The listing builds one solid part. Answer for the finished solid, in the listing's coordinates (mm). A direction names the side the tool comes from. Give positions to 0.01 mm unless a question says otherwise; leave off trailing zeros. Write each loop counter-clockwise with the first axis right and the second up, starting at its lowest first coordinate (ties: lowest second). Pieces come first, ordered by that corner, then holes. Notation, with made-up numbers: (44.25, 44) -> (92.25, 44) arc R18 cw to (92.25, 72) -> close; hole circle Ø3 at (69.5, 74). An arc over 180 degrees is marked (long way). Write each question's results on one line, items separated by ' | '. Start each with the question number.
from build123d import *

# Parameters (mm, degrees)
CUT_EXTRUDE2_DEPTH      = 20
CUT_EXTRUDE3_START      = -20
SKETCH8_R               = 5
CUT_EXTRUDE3_DEPTH      = 20
CUT_EXTRUDE4_DEPTH      = 43.426406871
CUT_EXTRUDE4_DEPTH_BACK = 43.426406871
SKETCH11_R              = 0.7
CUT_EXTRUDE5_DEPTH      = 30.669007398
SKETCH13_R              = 1.3
CUT_EXTRUDE6_DEPTH      = 4


with BuildPart() as part:
    # Sketch5 → Revolve2 (revolve)
    with BuildSketch(Plane.XY, mode=Mode.PRIVATE) as revolve2_sk:
        Polygon((-9.041219405, 20), (0, 20), (0, -20), (-9.041219405, -20), (-10, -19), (-10, -1), (-9.041219405, 0), (-10, 1), (-10, 19), align=None)
    revolve(revolve2_sk.sketch.rotate(Axis((0, -53.191489362, 0), (0, 1, 0)), 180), axis=Axis((0, -53.191489362, 0), (0, 1, 0)))

    # Sketch6 → Cut-Extrude2 (cut)
    with BuildSketch(Plane(origin=(0, -20, 0), x_dir=(-1, 0, 0), z_dir=(0, -1, 0))):
        with BuildLine():
            Line((-3, 4), (-3, -4))
            ThreePointArc((-3, -4), (0, -5), (3, -4))
            Line((3, -4), (3, 4))
            ThreePointArc((3, 4), (0, 5), (-3, 4))
        make_face()
    extrude(amount=-CUT_EXTRUDE2_DEPTH, mode=Mode.SUBTRACT)

    # Sketch8 → Cut-Extrude3 (cut)
    with BuildSketch(Plane(origin=(0, 20, 0), x_dir=(1, 0, 0), z_dir=(0, 1, 0)).offset(CUT_EXTRUDE3_START)):
        with Locations(Location((0, 0, 0), (0, 0, 306.869897646))):
            Circle(SKETCH8_R)
    extrude(amount=CUT_EXTRUDE3_DEPTH, mode=Mode.SUBTRACT)

    # Sketch9 → Cut-Extrude4 (cut, two sides: drawn at the far end of the back side and taken through both)
    with BuildSketch(Plane(origin=(0, 20, 0), x_dir=(1, 0, 0), z_dir=(0, 1, 0)).offset(-CUT_EXTRUDE4_DEPTH_BACK)):
        with BuildLine():
            Line((-0.5, -4.974937186), (-0.5, -10.403800493))
            ThreePointArc((-0.5, -10.403800493), (0, -10.415808404), (0.5, -10.403800493))
            Line((0.5, -10.403800493), (0.5, -4.974937186))
            ThreePointArc((0.5, -4.974937186), (0, -5), (-0.5, -4.974937186))
        make_face()
    extrude(amount=CUT_EXTRUDE4_DEPTH + CUT_EXTRUDE4_DEPTH_BACK, mode=Mode.SUBTRACT)

    # Sketch11 → Cut-Extrude5 (cut, through all)
    with BuildSketch(Plane(origin=(9.5, 0, 0), x_dir=(0, 0, -1), z_dir=(1, 0, 0))):
        with Locations(Location((-7.5, 15, 0), (0, 0, 90))):
            Circle(SKETCH11_R)
        with Locations(Location((-7.5, 5, 0), (0, 0, 90))):
            Circle(SKETCH11_R)
        with Locations(Location((-7.5, -5, 0), (0, 0, 90))):
            Circle(SKETCH11_R)
        with Locations(Location((-7.5, -15, 0), (0, 0, 90))):
            Circle(SKETCH11_R)
    extrude(amount=-CUT_EXTRUDE5_DEPTH, mode=Mode.SUBTRACT)

    # Sketch13 → Cut-Extrude6 (cut)
    with BuildSketch(Plane(origin=(9.5, 0, 0), x_dir=(0, 0, -1), z_dir=(1, 0, 0))):
        with Locations((-7.5, 15)):
            Circle(SKETCH13_R)
        with Locations((-7.5, 5)):
            Circle(SKETCH13_R)
        with Locations((-7.5, -5)):
            Circle(SKETCH13_R)
        with Locations((-7.5, -15)):
            Circle(SKETCH13_R)
    extrude(amount=-CUT_EXTRUDE6_DEPTH, mode=Mode.SUBTRACT)


solid = part.part
1. The mould has two halves that part along Z. Classify faces 5 (the flat face through (-0.5, 0, 7)), 6 (the cylindrical face through (3.04, 4.48, 7.97)): pulls with the +Z half, pulls with the -Z half, needs draft (parallel to the pull), parting line crosses it, or undercut.
2. Section C-C (y = -9) is taken. Write down the section's boundary in (x, z).
3. Consider probe 1 along Y at (x, z) = (-3.75, 7.5); probe 2 along Y at (x, z) = (6.55, 7.5); probe 3 along Z at (x, y) = (1.5, -15). Determine where each line is inside the solid, lowest interval first. Write a range as [from, to].
4. Section D-D (x = -4) is taken. Give the number of separate pieces and of enclosed holes in the cut face, then the cut area to 3 significant figures.
5. Each of these flat-tipped pins is pushed along its axis until it touches: pin 1 Ø0.8 at (y, z) = (-15, 7.5) entering from -X; pin 2 Ø2 at (y, z) = (-5, 7.5) entering from +X; pin 3 Ø1 at (x, y) = (7, -10) entering from +Z; pin 4 Ø4 at (y, z) = (-15, 7.5) entering from -X. Where does it stop, or does it pass through?
6. Section A-A (y = -15) is taken. Write down the section's boundary in (x, z).
7. A tool of negligible diameter and unlimited length cuts with its end or side. For faces 1 (the flat face through (0.5, 0, 8)), 2 (the flat face through (4, 0, 0)), 3 (the cylindrical face through (6.4, 15, 6.2)), 4 (the flat face through (3, -10, 0)), from which of +Z, -Z, +X, -X, +Y, -Y can it reach the whole face along a straight path? Write none if from no direction.
8. Section B-B (x = 0) is taken. Write down the section's boundary in (y, z), then the cut area to 3 significant figures.
Results:
1) face 5: needs draft | face 6: undercut
2) outline: (-3, -4) -> (-3, 4) arc R5 cw to (-0.5, 4.97) -> (-0.5, 9.99) arc R10 ccw (long way) to (0.5, 9.99) -> (0.5, 4.97) arc R5 cw to (3, 4) -> (3, -4) arc R5 cw to start
3) probe 1: y = [-20, -15.7], [-14.3, -5.7], [-4.3, 4.3], [5.7, 14.3], [15.7, 20] | probe 2: y = [-19.04, -16.3], [-13.7, -6.3], [-3.7, -0.96], [0.96, 3.7], [6.3, 13.7], [16.3, 19.04] | probe 3: z = [-9.89, -4.77], [4.77, 6.8], [8.2, 9.89]
4) separate pieces: 1 | enclosed holes: 4 | area: 603 mm²
5) pin 1: passes through | pin 2: stops at x = 5.5 | pin 3: stops at z = 7.6 | pin 4: stops at x = -8.35
6) outline: (-7.33, 6.8) arc R10 ccw (long way) to (7.85, 6.2) -> (5.5, 6.2) -> (5.5, 6.8) -> (0.5, 6.8) -> (0.5, 4.97) arc R5 cw to (3, 4) -> (3, -4) arc R5 cw to (-3, -4) -> (-3, 4) arc R5 cw to (-0.5, 4.97) -> (-0.5, 6.8) -> close; (-5.72, 8.2) -> (-0.5, 8.2) -> (-0.5, 9.99) arc R10 ccw to start; (0.5, 8.2) -> (5.5, 8.2) -> (5.5, 8.35) arc R10 ccw to (0.5, 9.99) -> close
7) face 1: +Z, +Y, -Y | face 2: +Y | face 3: +X | face 4: +Y, -Y
8) outline: (-20, -9.04) -> (-19, -10) -> (-1, -10) -> (0, -9.04) -> (1, -10) -> (19, -10) -> (20, -9.04) -> (20, -5) -> (-20, -5) -> close | area: 198 mm²
